Check sheet for the modelled part. Datum: model origin and axes. Units: mm. A direction names the side the tool comes from. Give positions to 0.01 mm unless a question says otherwise; leave off trailing zeros. Write each loop counter-clockwise with the first axis right and the second up, starting at its lowest first coordinate (ties: lowest second). Pieces come first, ordered by that corner, then holes. Notation, with made-up numbers: M 58,3.25 L 94,3.25 A14 ccw 94,13.25 Z; hole C 57.25,30.5 d1. An arc over 180 degrees is marked long. Write item = value, one per line. Start each with the question number.
1) Cross-section at A-A, the plane z = 3.5. Record the cut outline in (x, y) (3 decimals).
2) Cross-section at D-D, the plane z = 7. Record the cut outline in (x, y) (3 decimals), plus the area to 3 significant figures.
3) Cross-section at C-C, the plane y = 52. Record the cut outline in (x, z).
4) Go/stop test with flat-tipped pins: pin 1 (13.5 mm diameter, centred on y = 37.5, z = 9.5, fed in from -X); pin 2 (1 mm diameter, centred on y = 43.5, z = 26, fed in from +X). Record where each tip stops, or that it passes through.
5) Scan lines: line 1 along Y through (x, z) = (27.75, 12.75); line 2 along X through (y, z) = (57, 10); line 3 along Y through (x, z) = (18.5, 28). Record each from-to range of solid material in increasing order. Write a range as [from, to].
6) Access from +Z, -Z, +X, -X, +Y, -Y to the whole of each face (thin tool, end or side, straight path). Record for faces 5 (the flat face through (29.718, 15, 15)), 6 (the flat face through (28.829, 43, 15)), 7 (the cylindrical face through (18.24, 13.94, 10.36)), 8 (the flat face through (0.889, 42, 15)), 9 (the cylindrical face through (5.415, 59.637, 10.765)).
7) Mould release check, pull along X, two halves, no side actions. Record for faces 1 (the flat face through (20, 7, 19.812)), 2 (the flat face through (0, 14, 15)), 3 (the flat face through (15, 0, 15)), 4 (the conical face through (21.408, 10.979, 24.834)): released by +X, released by -X, zero draft, split by the parting line, or undercut.
8) Cross-section at B-B, the plane x = 23. Record the cut outline in (y, z).
```python
from build123d import *

# Parameters (mm, degrees)
BOSS_EXTRUDE1_DEPTH = 29.718
SKETCH3_R           = 9.525
BOSS_EXTRUDE2_DEPTH = 7.62


with BuildPart() as part:
    # Sketch1 → Boss-Extrude1 (new body)
    with BuildSketch(Plane.XY):
        Polygon((0, 0), (0, 29.21), (0.889, 29.21), (0.889, 55.88), (28.829, 55.88), (28.829, 29.21), (29.718, 29.21), (29.718, 0), align=None)
    extrude(amount=BOSS_EXTRUDE1_DEPTH)

    # Sketch3 → Boss-Extrude2 (add)
    with BuildSketch(Plane(origin=(0, 55.88, 0), x_dir=(1, 0, 0), z_dir=(0, 1, 0))):
        with Locations(Location((14.859, -9.525, 0), (0, 0, 90))):
            Circle(SKETCH3_R)
    extrude(amount=BOSS_EXTRUDE2_DEPTH)

    # Sketch13 → 1/4 NPT Tapped Hole1 (revolve, cut)
    with BuildSketch(Plane(origin=(14.859, 9.525, 29.718), x_dir=(0, -1, 0), z_dir=(1, 0, 0))):
        Polygon((0, 0), (0, 29.718), (6.1976, 29.718), (5.5626, 29.083), (5.5626, 9.906), (6.557984794, 9.906), (6.8545837, 0), align=None)
    revolve(axis=Axis((14.859, 9.525, 36.068), (0, 0, -1)), mode=Mode.SUBTRACT)


solid = part.part
```
Reply:
q1.outline = M 0,0 L 29.718,0 L 29.718,29.21 L 28.829,29.21 L 28.829,55.88 L 22.236,55.88 L 22.236,63.5 L 7.482,63.5 L 7.482,55.88 L 0.889,55.88 L 0.889,29.21 L 0,29.21 Z; hole C 14.859,9.525 d11.125
q2.outline = M 0,0 L 29.718,0 L 29.718,29.21 L 28.829,29.21 L 28.829,55.88 L 24.043,55.88 L 24.043,63.5 L 5.675,63.5 L 5.675,55.88 L 0.889,55.88 L 0.889,29.21 L 0,29.21 Z; hole C 14.859,9.525 d11.125
q2.area = 1,660 mm2
q3.outline = M 0.89,0 L 28.83,0 L 28.83,29.72 L 0.89,29.72 Z
q4.pin_1 = 0.89
q4.pin_2 = 28.83
q5.line_1 = [0, 55.88]
q5.line_2 = [5.35, 24.37]
q5.line_3 = [0, 3.78], [15.27, 55.88]
q6.face_5 = +Z, -Z, +X, +Y, -Y
q6.face_6 = +Z, -Z, +X, +Y
q6.face_7 = +Z, -Z
q6.face_8 = +Z, -Z, -X, +Y
q6.face_9 = +Y
q7.face_1 = undercut
q7.face_2 = released by -X
q7.face_3 = zero draft
q7.face_4 = undercut
q8.outline = M 0,0 L 55.88,0 L 55.88,4.58 L 63.5,4.58 L 63.5,14.47 L 55.88,14.47 L 55.88,29.72 L 0,29.72 Z
